Geometry: see drawing. Coordinates: mm, zero at the bounding-box minimum. A direction names the side the tool comes from. Round coordinates to 2 decimals unless told otherwise and drop trailing zeros. Loops run counter-clockwise (first coordinate to the right, second up) from the corner with the lowest first, then second, coordinate; pieces in that order, holes last. Notation, with made-up numbers: (85.5, 19) - (129.5, 19) arc R21 cw to (129.5, 25) - close; hole circle Ø4 at (-34, -21.75). An arc over 180 degrees is marked (long way). Use CSV: the item, a comma, the result in double quotes.
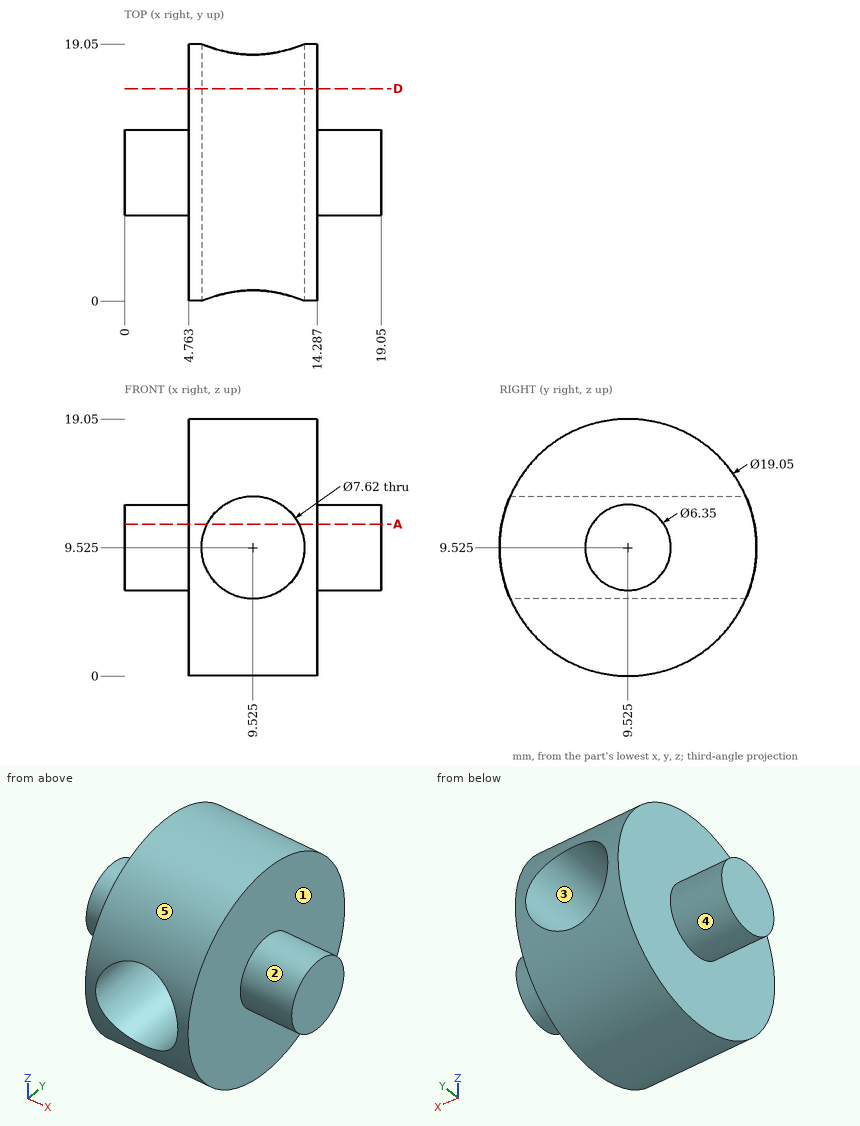
Item 1: Section A-A on z = 11.25. Return the cut outline in (x, y), plus the area to 3 significant figures.
Final values:
outline,"(0, 6.86) - (4.76, 6.86) - (4.76, 0.16) - (6.13, 0.16) - (6.13, 18.89) - (4.76, 18.89) - (4.76, 12.19) - (0, 12.19) - close; (12.92, 0.16) - (14.29, 0.16) - (14.29, 6.86) - (19.05, 6.86) - (19.05, 12.19) - (14.29, 12.19) - (14.29, 18.89) - (12.92, 18.89) - close"
area,"102 mm²"
Item 2: Pin query (flat end, axial travel): P1, Ø4, axis at x = 12.5, z = 15.5, coming from the +Y side; P2, Ø5, axis at x = 6.5, y = 17, coming from the +Z side; P3, Ø1, axis at y = 15, z = 9.5, coming from the +X side. Return the tip coordinate at first contact, or that it passes through.
Final values:
P1,"stops at y = 18.18"
P2,"stops at z = 17.65"
P3,"stops at x = 14.29"
Item 3: Mould query, pull axis Z, two halves, no side actions, for the marked faces 1, 2 and 3. Classes: released by +Z, released by -Z, zero draft, split by the parting line, or undercut.
Final values:
face 1,"zero draft"
face 2,"split by the parting line"
face 3,"undercut"
Item 4: Reachability of the marked faces 4 and 5 from +Z, -Z, +X, -X, +Y, -Y: full face, straight path, thin tool, end or side. Return the list, or none.
Final values:
face 4,"-X"
face 5,"+X, -X"
Item 5: Section D-D on y = 15.75. Return the cut outline in (x, z) (1 decimal).
Final values:
outline,"(4.8, 2.3) - (14.3, 2.3) - (14.3, 16.7) - (4.8, 16.7) - close; hole circle Ø7.6 at (9.5, 9.5)"
Item 6: Material intervals for line 1 (X direction, y = 15.75, z = 7) (1 decimal); line 2 (X direction, y = 5.5, z = 15.5); line 3 (X direction, y = 13.25, z = 10.25) (1 decimal), sorted ascending.
Final values:
line 1,"x = 4.8 to 6.7, 12.4 to 14.3"
line 2,"x = 4.76 to 14.29"
line 3,"x = 4.8 to 5.8, 13.3 to 14.3"
